Part model, mm, in its own coordinate system. Give positions to 0.01 mm unless a question says otherwise; leave off trailing zeros. Write each loop counter-clockwise with the first axis right and the second up, starting at its lowest first coordinate (ties: lowest second). Pieces come first, ordered by that corner, then holes.
from build123d import *

# Parameters (mm, degrees)
SKETCH1_R           = 1.6
BOSS_EXTRUDE1_DEPTH = 3
SKETCH2_W           = 25
SKETCH2_H           = 30.59
CUT_EXTRUDE1_DEPTH  = 39.14773912


with BuildPart() as part:
    # Sketch1 → Boss-Extrude1 (new body)
    with BuildSketch(Plane(origin=(0, 0, 0), x_dir=(1, 0, 0), z_dir=(0, 1, 0))):
        Polygon((-29.5, 24), (-29.5, 8), (-26.5, 8), (-26.5, -8), (-29.5, -8), (-29.5, -24), (-9.833333333, -24), (-9.833333333, -21), (9.833333333, -21), (9.833333333, -24), (29.5, -24), (29.5, -8), (26.5, -8), (26.5, 8), (29.5, 8), (29.5, 24), (9.833333333, 24), (9.833333333, 21), (-9.833333333, 21), (-9.833333333, 24), align=None)
        with Locations(Location((-21.0185, 15.69, 0), (0, 0, 270))):
            Circle(SKETCH1_R, mode=Mode.SUBTRACT)
        with Locations(Location((21.0185, 15.69, 0), (0, 0, 270))):
            Circle(SKETCH1_R, mode=Mode.SUBTRACT)
        with Locations(Location((21.0185, -13.52, 0), (0, 0, 270))):
            Circle(SKETCH1_R, mode=Mode.SUBTRACT)
    extrude(amount=BOSS_EXTRUDE1_DEPTH)

    # Sketch2 → Cut-Extrude1 (cut, through all)
    with BuildSketch(Plane(origin=(0, 3, 0), x_dir=(1, 0, 0), z_dir=(0, 1, 0))):
        with Locations((-12.5, -2.705)):
            Rectangle(SKETCH2_W, SKETCH2_H)
    extrude(amount=-CUT_EXTRUDE1_DEPTH, mode=Mode.SUBTRACT)


solid = part.part
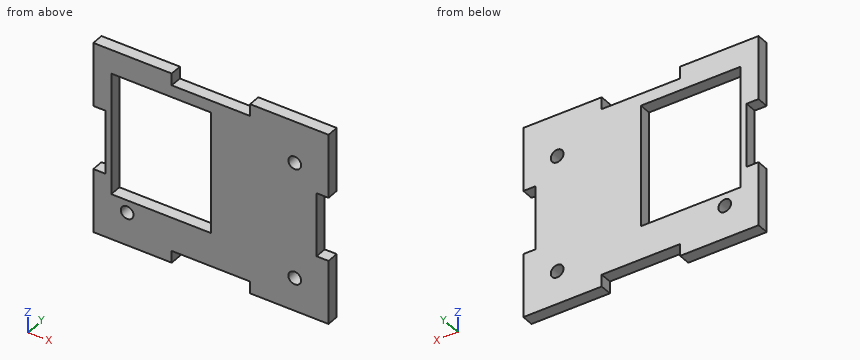
1) Flat gauge pin, fed straight in: P1, Ø1.5, axis at x = 4.5, y = 1.5, coming from the -Z side. Where does the tip first touch, or does it go through?
Check result:
P1: stops at z = -21
2) Saw through at B-B (z = 13.52). Write the cut outline in (x, y).
Check result:
outline: (-29.5, 0) - (-25, 0) - (-25, 3) - (-29.5, 3) - close; (0, 0) - (19.42, 0) - (19.42, 3) - (0, 3) - close; (22.62, 0) - (29.5, 0) - (29.5, 3) - (22.62, 3) - close
3) Drill centre lines: L1, parallel to X at y = 1.85, z = -15.69; L2, parallel to X at y = 2.7, z = 7; L3, parallel to Z at x = -12, y = 2.4. Where is each one in solid material? Low to high.
Check result:
L1: x = -29.5 to -22.62, -19.42 to 19.42, 22.62 to 29.5
L2: x = -26.5 to -25, 0 to 26.5
L3: z = -24 to -12.59, 18 to 24
4) Saw through at C-C (x = 22). Write the cut outline in (y, z).
Check result:
outline: (0, -24) - (3, -24) - (3, -16.95) - (0, -16.95) - close; (0, -14.43) - (3, -14.43) - (3, 12.26) - (0, 12.26) - close; (0, 14.78) - (3, 14.78) - (3, 24) - (0, 24) - close
5) Saw through at A-A (z = 5). Write the cut outline in (x, y), and give its area (3 significant figures).
Check result:
outline: (-26.5, 0) - (-25, 0) - (-25, 3) - (-26.5, 3) - close; (0, 0) - (26.5, 0) - (26.5, 3) - (0, 3) - close
area: 84.0 mm2
6) Saw through at D-D (z = -11). Write the cut outline in (x, y), and give its area (3 significant figures).
Check result:
outline: (-29.5, 0) - (-25, 0) - (-25, 3) - (-29.5, 3) - close; (0, 0) - (29.5, 0) - (29.5, 3) - (0, 3) - close
area: 102 mm2
